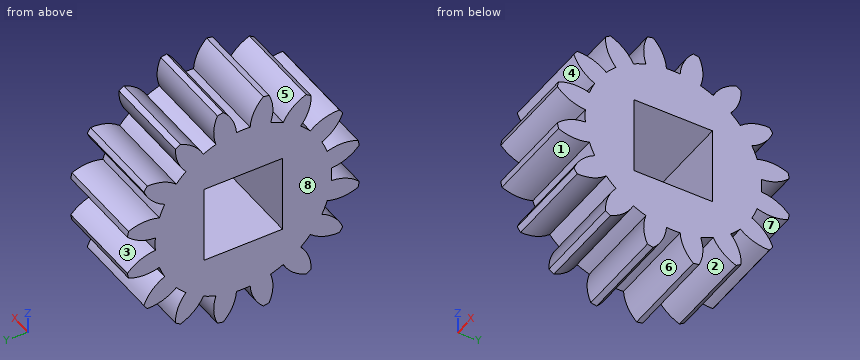
```python
from build123d import *

# Parameters (mm, degrees)
BASPROSKE_W        = 7
BASPROSKE_H        = 9
TOOTHCUT_DEPTH     = 15.525839046
TEETHCUTS_COUNT    = 16
BORSKE_R           = 3
BORE_DEPTH         = 50.0001016
SKETCH1_W          = 6
SKETCH1_H          = 6
CUT_EXTRUDE1_DEPTH = 10


with BuildPart() as part:
    # BasProSke → Base-Revolve (revolve)
    with BuildSketch(Plane(origin=(0, 0, 0), x_dir=(1, 0, 0), z_dir=(0, 1, 0)), mode=Mode.PRIVATE) as base_revolve_sk:
        with Locations((3.5, 4.5)):
            Rectangle(BASPROSKE_W, BASPROSKE_H)
    revolve(base_revolve_sk.sketch.rotate(Axis((-10, 0, 0), (1, 0, 0)), 180), axis=Axis((-10, 0, 0), (1, 0, 0)))

    # TooCutSke → ToothCut (cut, through all)
    with BuildSketch(Plane(origin=(0, 0, 0), x_dir=(0, 0, -1), z_dir=(1, 0, 0))):
        with BuildLine():
            ThreePointArc((0.523792937, 6.728643397), (0, 6.749), (-0.523792937, 6.728643397))
            ThreePointArc((-0.523792937, 6.728643397), (-0.828704482, 7.90962059), (-1.553355277, 8.890721711))
            ThreePointArc((-1.553355277, 8.890721711), (0, 9.0254), (1.553355277, 8.890721711))
            ThreePointArc((1.553355277, 8.890721711), (0.828704482, 7.90962059), (0.523792937, 6.728643397))
        make_face()
    toothcut = extrude(amount=TOOTHCUT_DEPTH, mode=Mode.SUBTRACT)

    # TeethCuts: ToothCut ×16 about axis
    teethcuts_axis = Axis((0, 0, 0), (1, 0, 0))
    for i in range(1, TEETHCUTS_COUNT):
        add(toothcut.rotate(teethcuts_axis, i * 360 / TEETHCUTS_COUNT), mode=Mode.SUBTRACT)

    # BorSke → Bore (cut, symmetric)
    with BuildSketch(Plane(origin=(0, 0, 0), x_dir=(0, 0, -1), z_dir=(1, 0, 0))):
        with Locations(Location((0, 0, 0), (0, 0, 180))):
            Circle(BORSKE_R)
    extrude(amount=BORE_DEPTH, both=True, mode=Mode.SUBTRACT)

    # Sketch1 → Cut-Extrude1 (cut)
    with BuildSketch(Plane(origin=(7, 0, 0), x_dir=(0, 0, -1), z_dir=(1, 0, 0))):
        Rectangle(SKETCH1_W, SKETCH1_H)
    extrude(amount=-CUT_EXTRUDE1_DEPTH, mode=Mode.SUBTRACT)


solid = part.part
```
Could you check a few things on this model? Use its own coordinates, in mm. Face numbers are marked on the shaded views. A direction names the side the tool comes from. Coordinates: 2 decimals unless noted, no trailing zeros. Order: outer loops, then holes, each group sorted by start corner. A loop starts at its lowest first (then second) coordinate and runs counter-clockwise, first axis right, second up. Notation, with made-up numbers: M 24,33 L 80,33 A24 ccw 80,68 Z; hole C -33,40.5 d7. An arc over 180 degrees is marked long. Use a Markdown table: item, result. Add a question column.
Q1. I'm going to push flat-ended pins straight in: pin 1 (1.8 mm diameter, centred on x = 3.5, y = 0, fed in from -Z); pin 2 (1.8 mm diameter, centred on x = 2.5, z = -1.5, fed in from -Y); pin 3 (1.5 mm diameter, centred on x = 2, z = 5, fed in from +Y). Where does each tip first touch, or does it pass through?
Q2. Which directions (+Z, -Z, +X, -X, +Y, -Y) give clear straight access to the entire face, cutting with the end or side of a thin tool? Please do the marked faces 1, 2, 3, 4 and 5.
Q3. I want a section at A-A on z = -1. List the corners of the cut face in (x, y) for me.
Q4. I want a section at D-D on y = -4. List the corners of the cut face in (x, z) for me.
Q5. If I drill on L1, parallel to Z at x = 6.75, y = -7; L2, parallel to Z at x = 4.5, y = -6.5; L3, parallel to Z at x = 2, y = -7.5, over which ranges is the centre line in solid material (lowest first)?
Q6. I want a section at C-C on z = 5.5. List the corners of the cut face in (x, y) for me.
Q7. I want a section at B-B on y = 2.5. List the corners of the cut face in (x, z) for me, then the cut area to 3 significant figures.
Q8. We'd pull the mould along Z, two halves only. Please class the marked faces 6, 7 and 8: pulls with the +Z half, pulls with the -Z half, needs draft (parallel to the pull), parting line crosses it, or undercut.
Checked values:
| question | item | result |
|---|---|---|
| 1 | pin 1 | z = -8.05 |
| 1 | pin 2 | y = -8.87 |
| 1 | pin 3 | y = 7.61 |
| 2 | face 1 | +X, -X |
| 2 | face 2 | -Z, +X, -X |
| 2 | face 3 | +X, -X, +Y |
| 2 | face 4 | +X, -X, -Y |
| 2 | face 5 | +Z, +X, -X |
| 3 | outline | M 0,-8.22 L 7,-8.22 L 7,-3 L 0,-3 Z; M 0,3 L 7,3 L 7,8.22 L 0,8.22 Z |
| 4 | outline | M 0,-7.16 L 7,-7.16 L 7,7.16 L 0,7.16 Z |
| 5 | L1 | -5.18 to -3.8, -2.23 to -0.55, 0.55 to 2.23, 3.8 to 5.18 |
| 5 | L2 | -5.1 to -3.35, -2.12 to 2.12, 3.35 to 5.1 |
| 5 | L3 | -4.97 to -4.55, -2.27 to -0.67, 0.67 to 2.27, 4.55 to 4.97 |
| 6 | outline | M 0,-4.67 L 7,-4.67 L 7,4.67 L 0,4.67 Z |
| 7 | outline | M 0,-6.27 L 7,-6.27 L 7,-3 L 0,-3 Z; M 0,3 L 7,3 L 7,6.27 L 0,6.27 Z |
| 7 | area | 45.8 mm² |
| 8 | face 6 | pulls with the -Z half |
| 8 | face 7 | undercut |
| 8 | face 8 | needs draft |
